Geometry: final body of the model. Coordinates: model frame, mm. Face numbers are marked on the shaded views. A direction names the side the tool comes from. Coordinates: 2 decimals unless noted, no trailing zeros. Order: outer loops, then holes, each group sorted by start corner. A loop starts at its lowest first (then second) coordinate and runs counter-clockwise, first axis right, second up. Notation, with made-up numbers: (47, 8.25) -> (71, 8.25) arc R15 cw to (71, 32.25) -> close; hole circle Ø1 at (-8, 57). An arc over 180 degrees is marked (long way). Use one line per item in the form item = value.
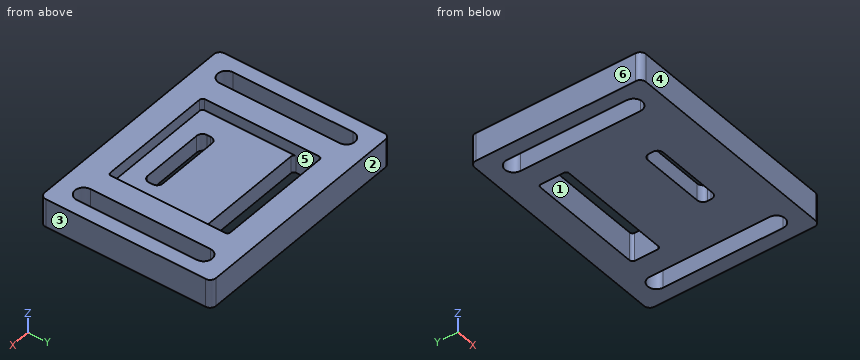
```python
from build123d import *

# Parameters (mm, degrees)
SCHIZZO2_W                   = 40
SCHIZZO2_H                   = 30
SCHIZZO2_W_2                 = 21
SCHIZZO2_H_2                 = 21
ESTRUSIONE_ESTRUSIONE1_DEPTH = 5
SCHIZZO2_3_W                 = 21
SCHIZZO2_3_H                 = 16
SCHIZZO2_3_W_2               = 13
SCHIZZO2_3_H_2               = 2.673538732
ESTRUSIONE_ESTRUSIONE2_DEPTH = 3
RACCORDO2_R                  = 1
RACCORDO3_R                  = 1
RACCORDO4_R                  = 0.5


with BuildPart() as part:
    # Schizzo2 → Estrusione-Estrusione1 (new body)
    with BuildSketch(Plane.XY):
        with Locations((20, 15)):
            Rectangle(SCHIZZO2_W, SCHIZZO2_H)
        with BuildLine():
            ThreePointArc((34.5, 4.5), (36, 3), (37.5, 4.5))
            Line((37.5, 4.5), (37.5, 25.5))
            ThreePointArc((37.5, 25.5), (36, 27), (34.5, 25.5))
            Line((34.5, 25.5), (34.5, 4.5))
        make_face(mode=Mode.SUBTRACT)
        with BuildLine():
            ThreePointArc((2.5, 4.5), (4, 3), (5.5, 4.5))
            Line((5.5, 4.5), (5.5, 25.5))
            ThreePointArc((5.5, 25.5), (4, 27), (2.5, 25.5))
            Line((2.5, 25.5), (2.5, 4.5))
        make_face(mode=Mode.SUBTRACT)
        with Locations((20, 15)):
            Rectangle(SCHIZZO2_W_2, SCHIZZO2_H_2, mode=Mode.SUBTRACT)
    extrude(amount=ESTRUSIONE_ESTRUSIONE1_DEPTH)

    # Schizzo2_3 → Estrusione-Estrusione2 (add)
    with BuildSketch(Plane.XY):
        with Locations((20, 12.5)):
            Rectangle(SCHIZZO2_3_W, SCHIZZO2_3_H)
        with Locations((20, 8.836769366)):
            Rectangle(SCHIZZO2_3_W_2, SCHIZZO2_3_H_2, mode=Mode.SUBTRACT)
    extrude(amount=ESTRUSIONE_ESTRUSIONE2_DEPTH)

    # Raccordo2
    raccordo2_edges = [part.edges().sort_by_distance(p)[0] for p in [
        (13.5, 10.173538732, 1.5),
        (26.5, 10.173538732, 1.5),
        (26.5, 7.5, 1.5),
        (13.5, 7.5, 1.5),
    ]]
    fillet(raccordo2_edges, radius=RACCORDO2_R)

    # Raccordo3
    raccordo3_edges = [part.edges().sort_by_distance(p)[0] for p in [
        (0, 0, 2.5),
        (0, 30, 2.5),
        (40, 30, 2.5),
        (40, 0, 2.5),
    ]]
    fillet(raccordo3_edges, radius=RACCORDO3_R)

    # Raccordo4
    raccordo4_edges = [part.edges().sort_by_distance(p)[0] for p in [
        (9.5, 25.5, 2.5),
        (9.5, 4.5, 4),
        (30.5, 4.5, 4),
        (30.5, 25.5, 2.5),
        (30.5, 20.5, 1.5),
        (9.5, 20.5, 1.5),
    ]]
    fillet(raccordo4_edges, radius=RACCORDO4_R)


solid = part.part
```
1) Material intervals for probe 1 along X at (y, z) = (18, 0.45); probe 2 along Y at (x, z) = (25.5, 1.5); probe 3 along X at (y, z) = (9, 0.2), sorted ascending. Write a range as from..to.
Results found:
probe_1 = 0..2.5, 5.5..34.5, 37.5..40
probe_2 = 0..7.5, 10.17..20.5, 25.5..30
probe_3 = 0..2.5, 5.5..13.5, 26.5..34.5, 37.5..40
2) Section A-A, the plane x = 11. Output: boundary loops of the cut face in (y, z), and give its area (3 significant figures).
Results found:
outline = (0, 0) -> (20.5, 0) -> (20.5, 3) -> (4.5, 3) -> (4.5, 5) -> (0, 5) -> close; (25.5, 0) -> (30, 0) -> (30, 5) -> (25.5, 5) -> close
area = 93.0 mm2
3) Section B-B, the plane y = 19.5. Output: boundary loops of the cut face in (x, z), and give its area (3 significant figures).
Results found:
outline = (0, 0) -> (2.5, 0) -> (2.5, 5) -> (0, 5) -> close; (5.5, 0) -> (34.5, 0) -> (34.5, 5) -> (30.5, 5) -> (30.5, 3) -> (9.5, 3) -> (9.5, 5) -> (5.5, 5) -> close; (37.5, 0) -> (40, 0) -> (40, 5) -> (37.5, 5) -> close
area = 128 mm2
4) Contact query for a flat-ended pin moving along its axis: P1, Ø1, axis at x = 19.5, y = 10, coming from the +Z side. Output: stop coordinate, or through.
Results found:
P1 = 3
5) Section C-C, the plane z = 2.2. Give the number of separate pieces and of enclosed holes in the cut face, and give its area (3 significant figures).
Results found:
separate_pieces = 1
enclosed_holes = 4
area = 920 mm2
6) Access query for the marked faces 5 and 6. Directions: +Z, -Z, +X, -X, +Y, -Y. A direction counts if a zero-diameter tool reaches every point of the face in a straight line with its end or side. Return the directions, or none.
Results found:
face_5 = +Z
face_6 = +Z, -Z, -X, +Y, -Y
7) Section D-D, the plane x = 22. Output: boundary loops of the cut face in (y, z), and give its area (3 significant figures).
Results found:
outline = (0, 0) -> (7.5, 0) -> (7.5, 3) -> (4.5, 3) -> (4.5, 5) -> (0, 5) -> close; (10.17, 0) -> (20.5, 0) -> (20.5, 3) -> (10.17, 3) -> close; (25.5, 0) -> (30, 0) -> (30, 5) -> (25.5, 5) -> close
area = 85.0 mm2
8) Pull-direction query (Y, two-part tool) for the marked faces 1, 2, 3 and 4; classes: released by +Y, released by -Y, zero draft, split by the parting line, or undercut.
Results found:
face_1 = undercut
face_2 = released by +Y
face_3 = zero draft
face_4 = released by -Y
